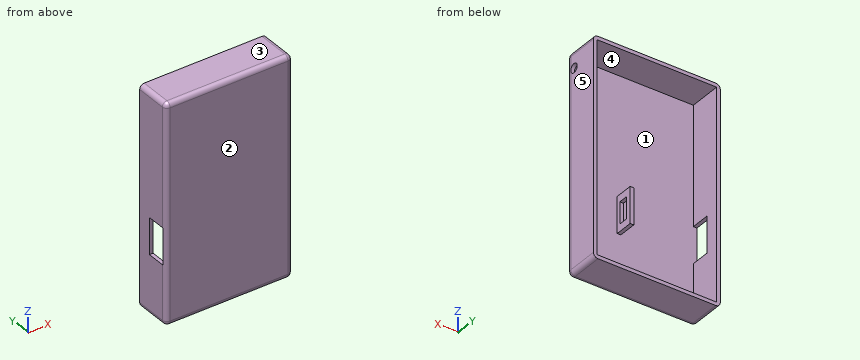
Autodesk Inventor part; units mm, degrees
ref_plane "YZ Plane" through (0, 0, 0) normal (1, 0, 0) x (0, 1, 0)
ref_plane "XZ Plane" through (0, 0, 0) normal (0, 1, 0) x (-1, 0, 0)
ref_plane "XY Plane" through (0, 0, 0) normal (0, 0, 1) x (1, 0, 0)
sketch "Sketch1" plane through (0, 0, 0) normal (0, 1, 0) x (-1, 0, 0)
  line L0 (0, 0) -> (88.9, 0)
  line L1 (88.9, 0) -> (88.9, -152.4)
  line L2 (88.9, -152.4) -> (0, -152.4)
  line L3 (0, -152.4) -> (0, 0)
  dimension "d0" = 88.9
  dimension "d1" = 152.4
extrude "Extrusion1" add sketch "Sketch1" along normal blind 25.4
shell "Shell1" thickness 2.54 removed faces 1 at (-59.2667, 25.4, -101.6)
sketch "Sketch2" plane through (-86.36, 2.54, -149.86) normal (1, 0, 0) x (0, 0, -1)
  point P0 (-149.86, -2.54)
sketch "Sketch7" plane through (0, 0, 0) normal (1, 0, 0) x (0, 0, -1)
  line L0 (152.4, 0) -> (0, 0)
  line L1 (0, 0) -> (0, 6.35)
  line L2 (0, 0) -> (0, 25.4)
  line L3 (0, 6.35) -> (12.7, 6.35)
  dimension "d21" = 6.35
  dimension "d22" = 12.7
  dimension "d23" = 90
hole "Hole1" at (0, 6.35, -12.7) direction (-1, 0, 0) diameter 6.35 depth 2.54 tip angle 118
fillet "Fillet2" radius 3.175 8 edges at (-44.45, 0, 0) (0, 12.7, 0) (0, 0, -76.2) (-88.9, 12.7, 0) (-88.9, 0, -76.2) (-44.45, 0, -152.4) (-88.9, 12.7, -152.4) (0, 12.7, -152.4)
sketch "Sketch9" plane through (-86.36, 2.54, -149.86) normal (1, 0, 0) x (0, 0, -1)
  line L0 (-0.635, 0.635) -> (-0.635, 22.86)
  line L1 (-0.635, 0.635) -> (-38.735, 0.635)
  line L2 (0, 0) -> (-147.32, 0)
  line L3 (-0.635, 0.635) -> (37.465, 0.635) construction
  line L4 (-38.735, 0.635) -> (-64.135, 0.635)
  line L5 (-64.135, 0.635) -> (-38.735, 0.635)
  line L6 (-38.735, 0.635) -> (-38.735, 13.335)
  line L7 (-38.735, 13.335) -> (-64.135, 13.335)
  line L8 (-64.135, 13.335) -> (-64.135, 0.635)
  point P0 (-149.86, -2.54)
  point P1 (-38.735, 0.635)
  dimension "d39" = 38.1
  dimension "d40" = 180
  dimension "d41" = 25.4
  dimension "d42" = 180
  dimension "d43" = 25.4
  dimension "d44" = 12.7
extrude "Extrusion7" cut sketch "Sketch9" against normal blind 5.08
sketch "Sketch10" plane through (-86.36, 2.54, -149.86) normal (1, 0, 0) x (0, 0, -1)
  line L0 (-38.735, 13.335) -> (-38.735, 0.635)
  line L1 (-38.735, 0.635) -> (-64.135, 0.635)
  line L2 (-64.135, 0.635) -> (-64.135, 0)
  line L3 (-64.135, 0) -> (-38.735, 0)
  line L4 (-38.735, 0) -> (-38.735, 0.635)
  point P0 (-149.86, -2.54)
  dimension "d47" = 25.4
  dimension "d48" = 0.635
extrude "Extrusion8" cut sketch "Sketch10" against normal blind 5.08
sketch "Sketch11" plane through (-86.36, 2.54, -149.86) normal (0, 1, 0) x (1, 0, 0)
  line L0 (0, -64.135) -> (-2.4759, -64.135)
  line L1 (0, -64.135) -> (50.8, -64.135)
  line L2 (0, -64.135) -> (50.8, -64.135) construction
  line L3 (50.8, -64.135) -> (53.34, -64.135)
  line L4 (53.34, -64.135) -> (53.34, -38.735)
  line L5 (53.34, -38.735) -> (50.8, -38.735)
  line L6 (50.8, -38.735) -> (50.8, -64.135)
  point P0 (86.36, -149.86)
  dimension "d51" = 50.8
  dimension "d52" = 0
  dimension "d53" = 2.54
  dimension "d54" = 25.4
extrude "Extrusion9" add sketch "Sketch11" along normal blind 12.7
sketch "Sketch12" plane through (-33.02, 2.54, -85.725) normal (1, 0, 0) x (0, 0, -1)
  line L0 (0, 0) -> (5.08, 0)
  line L1 (25.4, 0) -> (0, 0)
  line L2 (0, 0) -> (5.08, 0) construction
  line L3 (25.4, 0) -> (20.32, 0)
  line L4 (25.4, 0) -> (30.48, 0) construction
  line L5 (20.32, 0) -> (20.32, 2.54)
  line L6 (0, 0) -> (25.4, 0)
  line L7 (20.32, 0) -> (22.86, 0) construction
  line L8 (20.32, 2.54) -> (5.08, 2.54)
  line L9 (5.08, 2.54) -> (5.08, 8.89)
  line L10 (5.08, 8.89) -> (20.32, 8.89)
  line L11 (20.32, 8.89) -> (20.32, 2.54)
  point P0 (-85.725, -2.54)
  dimension "d57" = 5.08
  dimension "d58" = 0
  dimension "d59" = 5.08
  dimension "d60" = 180
  dimension "d61" = 2.54
  dimension "d62" = 90
  dimension "d63" = 15.24
  dimension "d64" = 6.35
extrude "Extrusion10" cut sketch "Sketch12" against normal blind 12.7
properties part number "OuterCase"
Verification items for the finished model (mm, model axes). Face numbers are marked on the shaded views. A direction names the side the tool comes from. Coordinates: 2 decimals unless noted, no trailing zeros. Order: outer loops, then holes, each group sorted by start corner. A loop starts at its lowest first (then second) coordinate and runs counter-clockwise, first axis right, second up. Notation, with made-up numbers: (58.25, 14.25) -> (65.25, 14.25) arc R23 ccw to (65.25, 22.25) -> close; hole circle Ø8 at (62, 24). An arc over 180 degrees is marked (long way). Put each result on its own line as item: value. Start each with the question number.
1) Release check for a two-part mould opening along Z. For the marked faces 1, 2 and 3 record: pulls with the +Z half, pulls with the -Z half, needs draft (parallel to the pull), parting line crosses it, or undercut.
2) Cross-section at C-C (z = -69.5). Enter the section's corners in (x, y), plus the area to 3 significant figures.
3) Tool access check on the marked faces 4 and 5. Record the directions out of +Z, -Z, +X, -X, +Y, -Y that give a thin tool (end or side, any length) a straight path to the whole face; none if there is none.
4) Cross-section at B-B (x = -67.5). Enter the section's corners in (y, z), plus the area to 3 significant figures.
5) Go/stop test with flat-tipped pins: pin 1 (2 mm diameter, centred on x = -34, z = -99.5, fed in from +Y); pin 2 (1.3 mm diameter, centred on x = -34, y = 7, fed in from +Z); pin 3 (4 mm diameter, centred on y = 9.5, z = -96, fed in from -X); pin 4 (5 mm diameter, centred on x = -42.5, z = -105, fed in from +Y). Record where each tip stops, or that it passes through.
6) Material ranges on L1, parallel to Z at x = -43.5, y = 24.5; L2, parallel to X at y = 23.25, z = -106; L3, parallel to X at y = 12.75, z = -97.5, recorded low to high.
Geometry check:
1. face 1: undercut
1. face 2: needs draft
1. face 3: pulls with the +Z half
2. outline: (-88.9, 3.17) arc R3.17 ccw to (-85.73, 0) -> (-3.17, 0) arc R3.17 ccw to (0, 3.17) -> (0, 25.4) -> (-2.54, 25.4) -> (-2.54, 2.54) -> (-86.36, 2.54) -> (-86.36, 25.4) -> (-88.9, 25.4) -> close
2. area: 338 mm^2
3. face 4: +Y
3. face 5: +Z, -Z, +X, +Y, -Y
4. outline: (0, -149.23) arc R3.17 ccw to (3.17, -152.4) -> (25.4, -152.4) -> (25.4, -149.86) -> (2.54, -149.86) -> (2.54, -2.54) -> (25.4, -2.54) -> (25.4, 0) -> (3.17, 0) arc R3.17 ccw to (0, -3.17) -> close
4. area: 499 mm^2
5. pin 1: stops at y = 15.24
5. pin 2: stops at z = 0
5. pin 3: stops at x = -35.56
5. pin 4: stops at y = 2.54
6. L1: z = -152.4 to -149.86, -2.54 to 0
6. L2: x = -88.9 to -86.36, -2.54 to 0
6. L3: x = -35.56 to -33.02, -2.54 to 0
